Work out the finished part from the listing and answer in its coordinate system (mm). A direction names the side the tool comes from. Give positions to 0.01 mm unless a question says otherwise; leave off trailing zeros. Loops run counter-clockwise (first coordinate to the right, second up) from the corner with the lowest first, then second, coordinate; pieces in that order, holes last. Notation, with made-up numbers: (-8.75, 58.5) - (45.25, 58.5) arc R20 ccw to (45.25, 88.5) - close; hole circle Ø1 at (-19, -18). An arc over 180 degrees is marked (long way). One line per question, with ' | ' between items. Start each with the question number.
1. For a pull along Z with two mould halves and no side action, classify faces 4 (the face through (-3.05, 3.08, -0.68)), 5 (the face through (2.045, 9, 0)), 6 (the face through (2.59, 30.71, 0.02)), 7 (the face through (0, 31.02, 0)) as released by +Z, released by -Z, zero draft, split by the parting line, or undercut.
2. Section B-B (y = 4) is taken. Determine the outline of the cut face in (x, z) (3 decimals), plus the area to 3 significant figures.
3. Find the intervals of material crossed by line 1 (Y direction, x = 2.75, z = 0); line 2 (Y direction, x = -1.75, z = -2.5); line 3 (Y direction, x = 2.75, z = 0.5), in increasing order.
4. Section C-C (y = 23) is taken. Determine the outline of the cut face in (x, z) (3 decimals), plus the area to 3 significant figures.
5. Each of these flat-tipped pins is pushed along its axis until it touches: pin 1 (0.6 mm diameter, centred on y = 7.5, z = 0, fed in from +X) (3 decimals); pin 2 (0.5 mm diameter, centred on x = 2.5, y = 8, fed in from +Z); pin 3 (1 mm diameter, centred on x = 2.5, y = 25, fed in from -Z). Where does it stop, or does it pass through?
6. Section A-A (z = 0) is taken. Determine the outline of the cut face in (x, y) (3 decimals), plus the area to 3 significant figures.
7. Which of the six approach directions +Z, -Z, +X, -X, +Y, -Y give full straight-line access (tool end or side, diameter ignored) to faces 1 (the face through (-2.938, 22.078, 0.117)), 2 (the face through (2.5, 26.1, -0.94)), 3 (the face through (-3.05, 30.58, -0.68))?
from build123d import *

# Parameters (mm, degrees)
SKETCH1_R           = 3.125
BOSS_EXTRUDE1_DEPTH = 31.02
SKETCH2_W           = 3.905114493
SKETCH2_H           = 0.39
SKETCH3_W           = 3.758921356
SKETCH3_H           = 0.39
SKETCH4_W           = 9.324870886
SKETCH4_H           = 0.39
SKETCH5_W           = 5.319059986
SKETCH5_H           = 0.39
CUT_EXTRUDE1_DEPTH  = 1.08
CUT_EXTRUDE2_DEPTH  = 1.08


with BuildPart() as part:
    # Sketch1 → Boss-Extrude1 (new body)
    with BuildSketch(Plane(origin=(0, 0, 0), x_dir=(1, 0, 0), z_dir=(0, 1, 0))):
        with Locations(Location((0, 0, 0), (0, 0, 270))):
            Circle(SKETCH1_R)
    extrude(amount=BOSS_EXTRUDE1_DEPTH)

    # Sketch2 → Cut-Revolve1 (revolve, cut)
    with BuildSketch(Plane(origin=(0, 0, 0), x_dir=(0, 0, -1), z_dir=(1, 0, 0))):
        with Locations((-4.892557247, 6.445)):
            Rectangle(SKETCH2_W, SKETCH2_H)
    revolve(axis=Axis((0, 10.072914163, 0), (0, -1, 0)), mode=Mode.SUBTRACT)

    # Sketch3 → Cut-Revolve2 (revolve, cut)
    with BuildSketch(Plane(origin=(0, 0, 0), x_dir=(0, 0, -1), z_dir=(1, 0, 0)), mode=Mode.PRIVATE) as cut_revolve2_sk:
        with Locations((-4.819460678, 11.835)):
            Rectangle(SKETCH3_W, SKETCH3_H)
    revolve(cut_revolve2_sk.sketch.rotate(Axis((0, 13.686668931, 0), (0, -1, 0)), 180), axis=Axis((0, 13.686668931, 0), (0, -1, 0)), mode=Mode.SUBTRACT)

    # Sketch4 → Cut-Revolve3 (revolve, cut)
    with BuildSketch(Plane(origin=(0, 0, 0), x_dir=(0, 0, -1), z_dir=(1, 0, 0)), mode=Mode.PRIVATE) as cut_revolve3_sk:
        with Locations((-7.602435443, 22.075)):
            Rectangle(SKETCH4_W, SKETCH4_H)
    revolve(cut_revolve3_sk.sketch.rotate(Axis((0, 25.014989783, 0), (0, -1, 0)), 180), axis=Axis((0, 25.014989783, 0), (0, -1, 0)), mode=Mode.SUBTRACT)

    # Sketch5 → Cut-Revolve4 (revolve, cut)
    with BuildSketch(Plane(origin=(0, 0, 0), x_dir=(0, 0, -1), z_dir=(1, 0, 0)), mode=Mode.PRIVATE) as cut_revolve4_sk:
        with Locations((-5.599529993, 29.965)):
            Rectangle(SKETCH5_W, SKETCH5_H)
    revolve(cut_revolve4_sk.sketch.rotate(Axis((0, 30.713823838, 0), (0, -1, 0)), 180), axis=Axis((0, 30.713823838, 0), (0, -1, 0)), mode=Mode.SUBTRACT)

    # Sketch6 → Cut-Extrude1 (cut)
    with BuildSketch(Plane(origin=(3.125, 0, 0), x_dir=(0, 0, -1), z_dir=(1, 0, 0))):
        with BuildLine():
            Line((0.94, 29.77), (0.94, 22.27))
            ThreePointArc((0.94, 22.27), (0, 21.33), (-0.94, 22.27))
            Line((-0.94, 22.27), (-0.94, 29.77))
            ThreePointArc((-0.94, 29.77), (0, 30.71), (0.94, 29.77))
        make_face()
    extrude(amount=-CUT_EXTRUDE1_DEPTH, mode=Mode.SUBTRACT)

    # Sketch7 → Cut-Extrude2 (cut)
    with BuildSketch(Plane(origin=(3.125, 0, 0), x_dir=(0, 0, -1), z_dir=(1, 0, 0))):
        with BuildLine():
            Line((0.94, 11.64), (0.94, 6.64))
            ThreePointArc((0.94, 6.64), (0, 5.7), (-0.94, 6.64))
            Line((-0.94, 6.64), (-0.94, 11.64))
            ThreePointArc((-0.94, 11.64), (0, 12.58), (0.94, 11.64))
        make_face()
    extrude(amount=-CUT_EXTRUDE2_DEPTH, mode=Mode.SUBTRACT)


solid = part.part
Conclusion:
1) face 4: split by the parting line | face 5: undercut | face 6: undercut | face 7: zero draft
2) outline: circle Ø6.25 at (0, 0) | area: 30.7 mm²
3) line 1: 0 to 5.7, 12.58 to 21.33, 30.71 to 31.02 | line 2: 0 to 6.25, 6.64 to 11.64, 12.03 to 21.88, 22.27 to 29.77, 30.16 to 31.02 | line 3: 0 to 5.84, 12.44 to 21.47, 30.57 to 31.02
4) outline: (2.045, -0.94) - (2.045, 0.94) - (2.98, 0.94) arc R3.125 ccw (long way) to (2.98, -0.94) - close | area: 28.7 mm²
5) pin 1: x = 2.045 | pin 2: z = 2.17 | pin 3: z = -2.4
6) outline: (-3.125, 0) - (3.125, 0) - (3.125, 5.7) - (2.045, 5.7) - (2.045, 12.58) - (3.125, 12.58) - (3.125, 21.33) - (2.045, 21.33) - (2.045, 30.71) - (3.125, 30.71) - (3.125, 31.02) - (-3.125, 31.02) - (-3.125, 30.16) - (-2.94, 30.16) - (-2.94, 29.77) - (-3.125, 29.77) - (-3.125, 22.27) - (-2.94, 22.27) - (-2.94, 21.88) - (-3.125, 21.88) - (-3.125, 12.03) - (-2.94, 12.03) - (-2.94, 11.64) - (-3.125, 11.64) - (-3.125, 6.64) - (-2.94, 6.64) - (-2.94, 6.25) - (-3.125, 6.25) - close | area: 176 mm²
7) face 1: none | face 2: +X | face 3: +Y, -Y
